Source: CAD feature listing. Evaluate the final solid. Frame: model axes, mm. A direction names the side the tool comes from. Round coordinates to 2 decimals unless told otherwise and drop trailing zeros. Order: outer loops, then holes, each group sorted by start corner. A loop starts at its lowest first (then second) coordinate and runs counter-clockwise, first axis right, second up. Notation, with made-up numbers: M -33.5,15.25 L 4.5,15.25 A18 cw 4.5,30.25 Z; hole C -36,33.5 d7. An arc over 180 degrees is marked long. Answer as CSV lines item,"result". Start each with the question number.
Item 1: Section query A-A on y = -2.5. Return the cut outline in (x, z).
Item 2: Section query C-C on z = 22. Return the cut outline in (x, y).
Item 3: Set-up query: faces 4 (the face through (-68, 17, 5)), 5 (the face through (-68, -16, 5)), 6 (the face through (-56, -25, 5)). Return all of +Z, -Z, +X, -X, +Y, -Y with unobstructed straight access to the full face (end or side cutting, diameter ignored); none if empty.
Item 4: Line query: line 1 (Z direction, x = -104, y = 4); line 2 (Y direction, x = -50, z = 7.75); line 3 (Y direction, x = -102.5, z = 37). Output: solid intervals per line, ascending. Write a range as [from, to].
Item 5: Section query B-B on x = -109. Return the cut outline in (y, z), plus the area to 3 significant figures.
Item 6: First-contact query: P1, Ø10, axis at y = 19, z = 7.5, coming from the +X side; P2, Ø12, axis at x = -59.5, y = 12, coming from the -Z side; P3, Ø8, axis at x = -82.5, z = 26, coming from the -Y side; P4, Ø2, axis at y = -5, z = 28.5, coming from the +X side. Flat tips, straight axial feed; report the tip coordinate or a pass-through.
Item 7: Pull-direction query (Y, two-part tool) for faces 1 (the face through (-55.99, -41.974, 4.93)), 2 (the face through (-124.476, -0.112, 30.046)), 3 (the face through (-6, 0, 5)); classes: +Y half, -Y half, draft (parallel to the pull), parting line (faces both ways), or undercut.
Item 8: Section query D-D on x = -50. Return the cut outline in (y, z).
from build123d import *

# Parameters (mm, degrees)
F0_R          = 6
F1_DEPTH      = 10
F2_R          = 10
F3_DEPTH      = 8
F3_DEPTH_BACK = 8


with BuildPart() as f1:
    # F0 (on Top) → F1 (new body)
    with BuildSketch(Plane.XY):
        with BuildLine():
            ThreePointArc((-35.6, -35.8), (-19.901005, -22.69799), (0, -18))
            ThreePointArc((0, -18), (18, 0), (0, 18))
            ThreePointArc((0, 18), (-19.959456, 23.374272), (-36.039548, 36.362472))
            ThreePointArc((-36.039548, 36.362472), (-56.029588, 41.960073), (-68, 25))
            Line((-68, 25), (-68, -25))
            ThreePointArc((-68, -25), (-55.6921, -42.076299), (-35.6, -35.8))
        make_face()
        with Locations((-50, -25)):
            Circle(F0_R, mode=Mode.SUBTRACT)
        Circle(F0_R, mode=Mode.SUBTRACT)
        with Locations((-50, 25)):
            Circle(F0_R, mode=Mode.SUBTRACT)
    extrude(amount=F1_DEPTH)

    # F2 (on Front) → F3 (join, two sides)
    with BuildSketch(Plane.XZ) as f3_sk:
        with BuildLine():
            ThreePointArc((-15, 10), (-54.838013, 18.269727), (-89.909731, 38.895689))
            ThreePointArc((-89.909731, 38.895689), (-124.684598, 29.493158), (-104, 0))
            Line((-104, 0), (-15, 0))
            Line((-15, 0), (-15, 10))
        make_face()
        with Locations((-104, 22)):
            Circle(F2_R, mode=Mode.SUBTRACT)
    extrude(amount=F3_DEPTH)
    extrude(f3_sk.sketch, amount=-F3_DEPTH_BACK)


solid = f1.part
Results:
1,outline,"M -104,0 L -5.45,0 L -5.45,10 L -15,10 A125 cw -89.91,38.9 A22 ccw long Z; M 5.45,0 L 17.83,0 L 17.83,10 L 5.45,10 Z; hole C -104,22 d20"
2,outline,"M -126,-8 L -114,-8 L -114,8 L -126,8 Z; M -94,-8 L -63.52,-8 L -63.52,8 L -94,8 Z"
3,face 4,"+Z, -Z, -X, +Y"
3,face 5,"+Z, -Z, -X, -Y"
3,face 6,"+Z, -Z"
4,line 1,"[0, 12], [32, 44]"
4,line 2,"[-43, -31], [-19, 19], [31, 43]"
4,line 3,"[-8, 8]"
5,outline,"M -8,0.58 L 8,0.58 L 8,13.34 L -8,13.34 Z; M -8,30.66 L 8,30.66 L 8,43.42 L -8,43.42 Z"
5,area,"408 mm^2"
6,P1,"x = 11.31"
6,P2,"z = 0"
6,P3,"y = -8"
6,P4,"x = -73.82"
7,face 1,"-Y half"
7,face 2,"draft"
7,face 3,"undercut"
8,outline,"M -43,0 L -31,0 L -31,10 L -43,10 Z; M -19,0 L 19,0 L 19,10 L 8,10 L 8,16.52 L -8,16.52 L -8,10 L -19,10 Z; M 31,0 L 43,0 L 43,10 L 31,10 Z"
